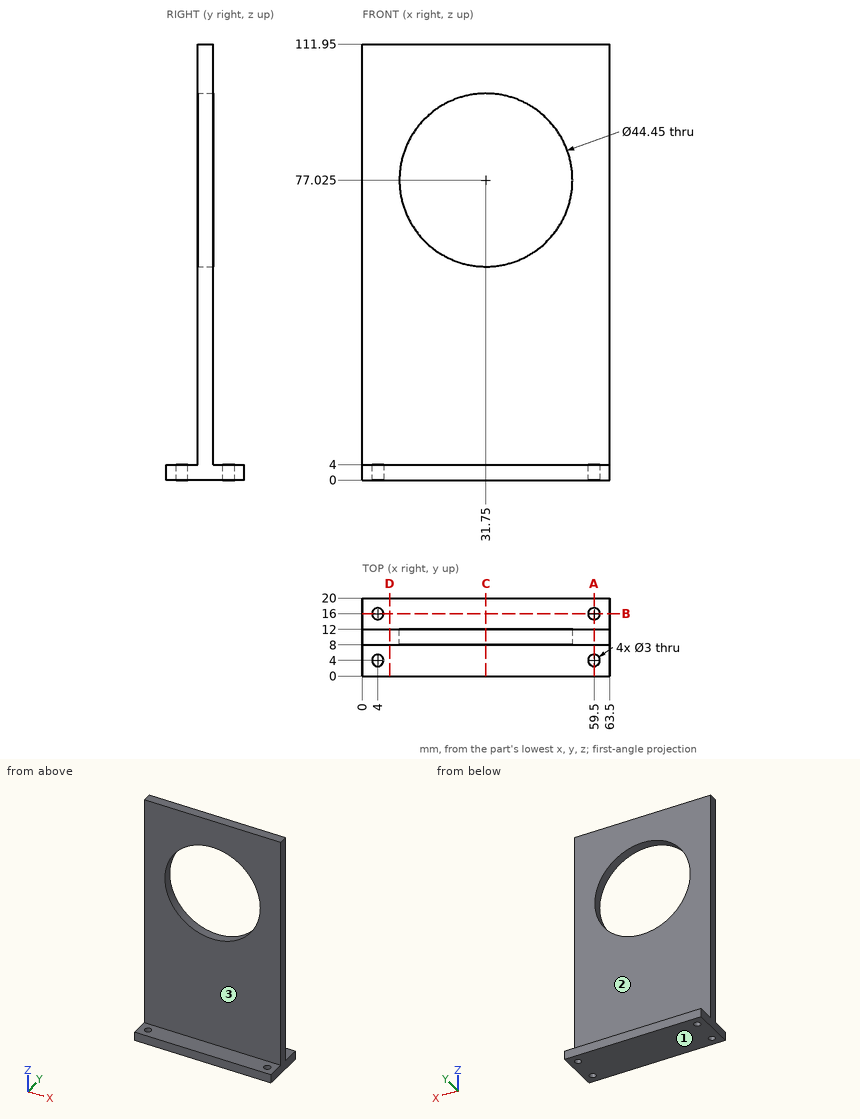
Study the drawing (mm; zero at the part's minimum x, y, z) and answer. A direction names the side the tool comes from. Give positions to 0.01 mm unless a question says otherwise; leave off trailing zeros. Loops run counter-clockwise (first coordinate to the right, second up) from the corner with the lowest first, then second, coordinate; pieces in that order, holes last. Notation, with made-up numbers: (-3.75, 58) -> (52.25, 58) arc R23 cw to (52.25, 71) -> close; hole circle Ø9 at (84, 64). An arc over 180 degrees is marked (long way). Write item = value, one per line. Start each with the question number.
(1) Given pin 1 Ø4 at (x, z) = (53.5, 73.5) entering from +Y; pin 2 Ø9 at (x, y) = (45, 17) entering from +Z, each flat-ended and moving along its own axis, determine where each tip first touches the part or whether it passes through.
(2) Find section D-D on x = 7. Give the vertices of the cut face in (y, z), and give its area (3 significant figures).
(3) Find section A-A on x = 59.5. Give the vertices of the cut face in (y, z), and give its area (3 significant figures).
(4) Which of the six approach directions +Z, -Z, +X, -X, +Y, -Y give full straight-line access (tool end or side, diameter ignored) to the marked faces 1, 2 and 3?
(5) Find section C-C on x = 31.75. Give the vertices of the cut face in (y, z), and give its area (3 significant figures).
(6) Find section B-B on y = 16. Give the vertices of the cut face in (x, z), and give its area (3 significant figures).
(7) Find the intervals of material crossed by probe 1 along Y at (x, z) = (59.5, 2.65); probe 2 along Z at (x, y) = (26, 19.25); probe 3 along Y at (x, z) = (28.5, 41), in increasing order. Write a range as from..to.
From the geometry:
q1.pin_1 = 12
q1.pin_2 = 4
q2.outline = (0, 0) -> (20, 0) -> (20, 4) -> (12, 4) -> (12, 111.95) -> (8, 111.95) -> (8, 4) -> (0, 4) -> close
q2.area = 512 mm^2
q3.outline = (0, 0) -> (2.5, 0) -> (2.5, 4) -> (0, 4) -> close; (5.5, 0) -> (14.5, 0) -> (14.5, 4) -> (12, 4) -> (12, 111.95) -> (8, 111.95) -> (8, 4) -> (5.5, 4) -> close; (17.5, 0) -> (20, 0) -> (20, 4) -> (17.5, 4) -> close
q3.area = 488 mm^2
q4.face_1 = -Z, +X, -X, +Y, -Y
q4.face_2 = +Z, +X, -X, +Y
q4.face_3 = +Z, +X, -X, -Y
q5.outline = (0, 0) -> (20, 0) -> (20, 4) -> (12, 4) -> (12, 54.8) -> (8, 54.8) -> (8, 4) -> (0, 4) -> close; (8, 99.25) -> (12, 99.25) -> (12, 111.95) -> (8, 111.95) -> close
q5.area = 334 mm^2
q6.outline = (0, 0) -> (2.5, 0) -> (2.5, 4) -> (0, 4) -> close; (5.5, 0) -> (58, 0) -> (58, 4) -> (5.5, 4) -> close; (61, 0) -> (63.5, 0) -> (63.5, 4) -> (61, 4) -> close
q6.area = 230 mm^2
q7.probe_1 = 0..2.5, 5.5..14.5, 17.5..20
q7.probe_2 = 0..4
q7.probe_3 = 8..12
